Model file for the job. Use its own axes, mm. A direction names the side the tool comes from. Give positions to 0.01 mm unless a question says otherwise; leave off trailing zeros. Write each loop counter-clockwise with the first axis right and the second up, starting at its lowest first coordinate (ties: lowest second). Pieces come first, ordered by that corner, then holes. Notation, with made-up numbers: (83.25, 61.25) - (95.25, 61.25) arc R11 cw to (95.25, 70.25) - close; hole circle Ø5 at (82.25, -39). An arc over 180 degrees is marked (long way). One line per item, written item: value. Start each with the question number.
(1) Cut at D-D, the plane y = 16.25. List the corners of the cut face in (x, z).
(2) Cut at C-C, the plane z = -4.25. List the corners of the cut face in (x, y).
(3) Mould opens along Y. For faces 4 (the face through (-7.585, 5.088, -12.948)), 5 (the face through (-6, 0, -7)), 6 (the face through (-5, 20, -5.689)) say: pulls with the +Y half, pulls with the -Y half, needs draft (parallel to the pull), parting line crosses it, or undercut.
(4) 3-axis set-ups, long thin cutter, end or side, ignore diameter. For faces 1 (the face through (-10, 11, -5)), 2 (the face through (-7, 10, -10)), 3 (the face through (-6.1, 4.9, -13.1)): which of +Z, -Z, +X, -X, +Y, -Y reach the whole face in a straight line?
(5) Cut at A-A, the plane y = 6.25. List the corners of the cut face in (x, z).
(6) Drop flat-ended pins along their axis: P1, Ø6, axis at x = -3.5, z = -8, coming from the -Y side; P2, Ø3, axis at x = -4.5, y = 17.5, coming from the -Z side; P3, Ø1, axis at x = -6, z = -4, coming from the +Y side; P4, Ø2, axis at y = 4.5, z = -13, coming from the +X side. Give the stop position or say it passes through.
(7) Cut at B-B, the plane x = -5. List the corners of the cut face in (y, z).
(8) Probe L1, parallel to Z at x = -5, y = 15; L2, parallel to Y at x = -5.75, z = -10.5; L3, parallel to Z at x = -8, y = 18.5. List the from-to ranges inside material, lowest first.
Autodesk Inventor part; units mm, degrees
ref_plane "YZ Plane" through (0, 0, 0) normal (1, 0, 0) x (0, 1, 0)
ref_plane "XZ Plane" through (0, 0, 0) normal (0, 1, 0) x (-1, 0, 0)
ref_plane "XY Plane" through (0, 0, 0) normal (0, 0, 1) x (1, 0, 0)
sketch "Sketch1" plane through (0, 0, 0) normal (0, 1, 0) x (-1, 0, 0)
  line L0 (0, -5.6886) -> (6.7556, -12.4442)
  line L1 (6.7556, -12.4442) -> (5.3414, -13.8584)
  line L2 (9.5, -18.017) -> (5.3414, -13.8584)
  line L3 (10, -18.017) -> (9.5, -18.017)
  line L4 (10, -18.017) -> (10, 0)
  line L5 (0, 0) -> (10, 0)
  line L6 (0, 0) -> (0, -5.6886)
  circle A0 centre (5, -2.8443) radius 1.339
extrude "Extrusion1" add sketch "Sketch1" along normal blind 10
sketch "Sketch2" plane through (0, 10, 0) normal (0, 1, 0) x (1, 0, 0)
  line L0 (0, 5.6886) -> (-10, 5.6886)
  line L1 (-10, 5.6886) -> (-10, 0)
  line L2 (-10, 0) -> (0, 0)
  line L3 (0, 0) -> (0, 5.6886)
extrude "Extrusion2" add sketch "Sketch2" along normal blind 20
sketch "Sketch3" plane through (0, 0, 0) normal (0, -1, 0) x (1, 0, 0)
  circle A0 centre (-5, -2.8443) radius 1.339
hole "Hole1" at (-5, 0, -2.8443) direction (0, 1, 0) diameter 4.318 depth 31 tip angle 118
sketch "Sketch4" plane through (-9.5, 0, -18.017) normal (0.7071, 0, -0.7071) x (-0.7071, 0, -0.7071)
  circle A0 centre (-2.9406, 5) radius 2.55
  point P0 (-19.4575, 0)
  dimension "d11" = 5.1
extrude "Extrusion3" cut sketch "Sketch4" against normal blind 0.1
sketch "Sketch5" plane through (-7.4914, 5, -15.867) normal (0.7071, 0, -0.7071) x (-0.7071, 0, -0.7071)
  circle A0 centre (0, 0) radius 2
  point P0 (-16.5169, -5)
  dimension "d15" = 4
extrude "Extrusion4" cut sketch "Sketch5" against normal blind 10
sketch "Sketch6" plane through (-9.5, 0, -18.017) normal (0.7071, 0, -0.7071) x (-0.7071, 0, -0.7071)
  circle A0 centre (-2.9406, 5) radius 2.55
  line L0 (-5.8811, 0) -> (0, 0)
  line L1 (0, 0) -> (0, 10)
  line L2 (-5.8811, 10) -> (0, 10)
  line L3 (-5.8811, 0) -> (-5.8811, 10)
  point P0 (-19.4575, 0)
hole "Hole2" at (-7.3787, 1.3, -15.8957) direction (-0.7071, 0, 0.7071) diameter 1.778 depth 8 tip angle 118
hole "Hole3" at (-7.3787, 8.7, -15.8957) direction (-0.7071, 0, 0.7071) diameter 1.778 depth 8 tip angle 118
properties part number "recessedCoverslip_v1"
Answers follow:
1. outline: (-10, -5.69) - (0, -5.69) - (0, 0) - (-10, 0) - close; hole circle Ø4.32 at (-5, -2.84)
2. outline: (-10, 0) - (-6.64, 0) - (-6.64, 30) - (-10, 30) - close; (-3.36, 0) - (0, 0) - (0, 30) - (-3.36, 30) - close
3. face 4: undercut
3. face 5: pulls with the -Y half
3. face 6: needs draft
4. face 1: +Z, -Z, -X, +Y, -Y
4. face 2: -Z, +X, -X, +Y
4. face 3: +X, +Y, -Y
5. outline: (-10, -18.02) - (-9.5, -18.02) - (-8.99, -17.51) - (-9.06, -17.44) - (-8.6, -16.97) - (-10, -15.57) - close; (-10, -11.15) - (-6.39, -14.76) - (-5.92, -14.29) - (-5.85, -14.37) - (-5.34, -13.86) - (-6.76, -12.44) - (0, -5.69) - (0, 0) - (-10, 0) - close; hole circle Ø4.32 at (-5, -2.84)
6. P1: stops at y = 0
6. P2: stops at z = -5.69
6. P3: passes through
6. P4: stops at x = -5.34
7. outline: (0, -10.69) - (10, -10.69) - (10, -5.69) - (30, -5.69) - (30, -5) - (0, -5) - close; (0, -0.69) - (30, -0.69) - (30, 0) - (0, 0) - close
8. L1: z = -5.69 to -5, -0.69 to 0
8. L2: y = 0 to 10
8. L3: z = -5.69 to 0
